```python
from build123d import *

# Parameters (mm, degrees)
F0_R     = 35.56
F0_R_2   = 4.3307
F1_DEPTH = 2.032
F2_R     = 18.9865
F3_DEPTH = 4.7625
F4_R     = 15.0749
F5_DEPTH = 6.7945


with BuildPart() as f1:
    # F0 (on Top) → F1 (new body)
    with BuildSketch(Plane.XY):
        Circle(F0_R)
        with Locations((-21.623095, -12.4841)):
            Circle(F0_R_2, mode=Mode.SUBTRACT)
        with Locations((21.623095, -12.4841)):
            Circle(F0_R_2, mode=Mode.SUBTRACT)
        with Locations((0, 24.9682)):
            Circle(F0_R_2, mode=Mode.SUBTRACT)
    extrude(amount=F1_DEPTH)

    # F2 (on face) → F3 (join)
    with BuildSketch(Plane.XY.offset(2.032)):
        Circle(F2_R)
    extrude(amount=F3_DEPTH)

    # F4 (on face) → F5 (cut, through all)
    with BuildSketch(Plane.XY.offset(6.7945)):
        Circle(F4_R)
    extrude(amount=-F5_DEPTH, mode=Mode.SUBTRACT)


solid = f1.part
```
Part model, mm, in its own coordinate system. A direction names the side the tool comes from. Round coordinates to 2 decimals unless told otherwise and drop trailing zeros. Write each loop counter-clockwise with the first axis right and the second up, starting at its lowest first coordinate (ties: lowest second). Pieces come first, ordered by that corner, then holes. Notation, with made-up numbers: M 83,65 L 123,65 A24 cw 123,98 Z; hole C -21,-3 d1. An arc over 180 degrees is marked long. Answer as CSV lines item,"result". Start each with the question number.
1) Band-saw the part on D-D (z = 3). List the corners of the cut face in (x, y), then the cut area to 3 significant figures.
2) Band-saw the part on B-B (y = -11.5). List the corners of the cut face in (x, z), then the cut area to 3 significant figures.
3) Band-saw the part on A-A (x = 0). List the corners of the cut face in (y, z), then the cut area to 3 significant figures.
4) Mould opens along X. For faces 3 (the face through (-6, 14, 6.794)), 4 (the face through (-7.709, -34.714, 1.002)), 5 (the face through (-3.268, -14.716, 3.445)) say: +X half, -X half, draft (parallel to the pull), parting line (faces both ways), or undercut.
5) Band-saw the part on C-C (y = 0). List the corners of the cut face in (x, z), then the cut area to 3 significant figures.
6) Drill centre lines: L1, parallel to Y at x = 0, z = 0.95; L2, parallel to Y at x = 0, z = 4; L3, parallel to X at y = -15.5, z = 2. Where is each one in solid material? Low to high.
7) Drop flat-ended pins along their axis: pin 1 (2 mm diameter, centred on x = 17.5, y = -14, fed in from +Z); pin 2 (1 mm diameter, centred on x = -16.5, z = 5, fed in from +Y); pin 3 (1 mm diameter, centred on x = 5.5, z = 5, fed in from -Y). Give the stop position or say it passes through.
8) Which spindle directions (+Z, -Z, +X, -X, +Y, -Y) get a long thin tool onto all of the face, cutting with end or side? Do faces 1 (the face through (25.754, -11.183, 1.002)), 2 (the face through (18.11, 5.7, 4.38)). Say none if no direction does.
Worked out:
1,outline,"C 0,0 d37.97; hole C 0,0 d30.15"
1,area,"419 mm²"
2,outline,"M -33.65,0 L -25.84,0 L -25.84,2.03 L -33.65,2.03 Z; M -17.41,0 L -9.75,0 L -9.75,6.79 L -15.11,6.79 L -15.11,2.03 L -17.41,2.03 Z; M 9.75,0 L 17.41,0 L 17.41,2.03 L 15.11,2.03 L 15.11,6.79 L 9.75,6.79 Z; M 25.84,0 L 33.65,0 L 33.65,2.03 L 25.84,2.03 Z"
2,area,"114 mm²"
3,outline,"M -35.56,0 L -15.07,0 L -15.07,6.79 L -18.99,6.79 L -18.99,2.03 L -35.56,2.03 Z; M 15.07,0 L 20.64,0 L 20.64,2.03 L 18.99,2.03 L 18.99,6.79 L 15.07,6.79 Z; M 29.3,0 L 35.56,0 L 35.56,2.03 L 29.3,2.03 Z"
3,area,"103 mm²"
4,face 3,"draft"
4,face 4,"parting line"
4,face 5,"undercut"
5,outline,"M -35.56,0 L -15.07,0 L -15.07,6.79 L -18.99,6.79 L -18.99,2.03 L -35.56,2.03 Z; M 15.07,0 L 35.56,0 L 35.56,2.03 L 18.99,2.03 L 18.99,6.79 L 15.07,6.79 Z"
5,area,"121 mm²"
6,L1,"-35.56 to -15.07, 15.07 to 20.64, 29.3 to 35.56"
6,L2,"-18.99 to -15.07, 15.07 to 18.99"
6,L3,"-32 to -24.73, -18.52 to 18.52, 24.73 to 32"
7,pin 1,"z = 2.03"
7,pin 2,"y = 10.22"
7,pin 3,"y = -18.32"
8,face 1,"+Z, -Z"
8,face 2,"+Z"
